Can you work these out from the model? Positions are in its coordinate system, mm. Face numbers are marked on the shaded views. A direction names the side the tool comes from. Coordinates: 2 decimals unless noted, no trailing zeros. Order: outer loops, then holes, each group sorted by start corner. A loop starts at its lowest first (then second) coordinate and runs counter-clockwise, first axis right, second up. Notation, with made-up numbers: (65, 40) - (74, 40) arc R29 ccw to (74, 61) - close; hole circle Ø5 at (-36, 60.5). An arc over 180 degrees is marked (long way). Use a Markdown table: item, result. Add a question column.
(1) I want a section at D-D (x = 0). List the corners of the cut face in (y, z) for me (1 decimal).
(2) I want a section at C-C (x = 10). List the corners of the cut face in (y, z) for me.
(3) I want a section at B-B (z = -2). State how many separate pieces and enclosed holes the cut face has, and give its area (3 significant figures).
(4) If I drill on L1, parallel to Y at x = 0, z = 3.75 (1 decimal); L2, parallel to X at y = 0.5, z = 2 (1 decimal); L3, parallel to Y at x = 0, z = -5.25 (3 decimals), over which ranges is the centre line in solid material (lowest first)? Write a range as [from, to].
(5) We'd pull the mould along X, two halves only. Please class the marked faces 1, 2 and 3: pulls with the +X half, pulls with the -X half, needs draft (parallel to the pull), parting line crosses it, or undercut.
(6) For pin 1 Ø5 at (x, z) = (7, -2.5) entering from -Y; pin 2 Ø1.4 at (x, y) = (-0.5, -9.5) entering from +Z; pin 3 Ø3.5 at (x, y) = (9.31, 0) entering from +Z; pin 4 Ø1 at (y, z) = (-8, -4) entering from -X, each with a flat end and sliding along its axis, tell me the tip position at first contact or that it passes through.
(7) On a 3-axis mill with a long thin cutter (end or side, diameter ignored), from which of +Z, -Z, +X, -X, +Y, -Y can I reach the whole of each face in a straight line? I mean the marked faces 4, 5 and 6. Say none if no direction works.
(8) I want a section at A-A (x = -3.5). List the corners of the cut face in (y, z) for me (3 decimals).
```python
from build123d import *

# Parameters (mm, degrees)
SKETCH1_R           = 12.5
BOSS_EXTRUDE1_DEPTH = 7.5
CUT_EXTRUDE3_REACH  = 25.184
SKETCH8_W           = 12.25
SKETCH8_H           = 12.25
SKETCH9_R           = 1.45
CUT_EXTRUDE4_DEPTH  = 10
FILLET1_R           = 1


with BuildPart() as part:
    # Sketch1 → Boss-Extrude1 (new, symmetric)
    with BuildSketch(Plane.XY):
        Circle(SKETCH1_R)
    extrude(amount=BOSS_EXTRUDE1_DEPTH, both=True)

    # Sketch8 → Cut-Extrude3 (cut, up to next)
    with BuildSketch(Plane.XY.offset(7.5), mode=Mode.PRIVATE) as cut_extrude3_sk1:
        Rectangle(SKETCH8_W, SKETCH8_H)
    cut_extrude3_tool1 = extrude(cut_extrude3_sk1.sketch, amount=-CUT_EXTRUDE3_REACH, mode=Mode.PRIVATE) & part.part
    add(cut_extrude3_tool1.solids().sort_by_distance((0, 0, 7.5))[0], mode=Mode.SUBTRACT)

    # Sketch9 → Cut-Extrude4 (cut)
    with BuildSketch(Plane.XY.offset(7.5)):
        with Locations((9.3125, 0)):
            Circle(SKETCH9_R)
        with Locations((0, -9.2875)):
            Circle(SKETCH9_R)
        with Locations((-9.2875, 0.025)):
            Circle(SKETCH9_R)
        with Locations((0.025, 9.3125)):
            Circle(SKETCH9_R)
    extrude(amount=-CUT_EXTRUDE4_DEPTH, mode=Mode.SUBTRACT)

    # Fillet1
    fillet1_edges = [part.edges().sort_by_distance(p)[0] for p in [
        (6.125, 6.125, 0),
        (6.125, -6.125, 0),
        (-6.125, -6.125, 0),
        (-6.125, 6.125, 0),
    ]]
    fillet(fillet1_edges, radius=FILLET1_R)


solid = part.part
```
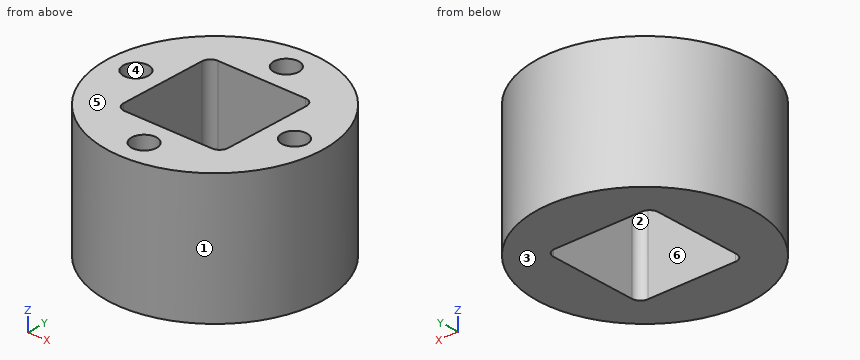
Answers follow:
| question | item | result |
|---|---|---|
| 1 | outline | (-12.5, -7.5) - (-6.1, -7.5) - (-6.1, 7.5) - (-7.8, 7.5) - (-7.8, -2.5) - (-10.7, -2.5) - (-10.7, 7.5) - (-12.5, 7.5) - close; (6.1, -7.5) - (12.5, -7.5) - (12.5, 7.5) - (10.8, 7.5) - (10.8, -2.5) - (7.9, -2.5) - (7.9, 7.5) - (6.1, 7.5) - close |
| 2 | outline | (-7.5, -7.5) - (7.5, -7.5) - (7.5, 7.5) - (1.28, 7.5) - (1.28, -2.5) - (-1.28, -2.5) - (-1.28, 7.5) - (-7.5, 7.5) - close |
| 3 | separate pieces | 1 |
| 3 | enclosed holes | 5 |
| 3 | area | 315 mm² |
| 4 | L1 | y = [-12.5, -10.7], [-7.8, -6.1], [6.1, 7.9], [10.8, 12.5] |
| 4 | L2 | x = [-12.5, -10.7], [-7.9, -6.1], [6.1, 8], [10.7, 12.5] |
| 4 | L3 | y = [-12.5, -6.125], [6.125, 12.5] |
| 5 | face 1 | parting line crosses it |
| 5 | face 2 | undercut |
| 5 | face 3 | needs draft |
| 6 | pin 1 | stops at y = -11.66 |
| 6 | pin 2 | stops at z = -2.5 |
| 6 | pin 3 | stops at z = 7.5 |
| 6 | pin 4 | stops at x = -10 |
| 7 | face 4 | +Z |
| 7 | face 5 | +Z, +X, -X, +Y, -Y |
| 7 | face 6 | +Z, -Z |
| 8 | outline | (-12, -7.5) - (-6.125, -7.5) - (-6.125, 7.5) - (-12, 7.5) - close; (6.125, -7.5) - (12, -7.5) - (12, 7.5) - (6.125, 7.5) - close |
